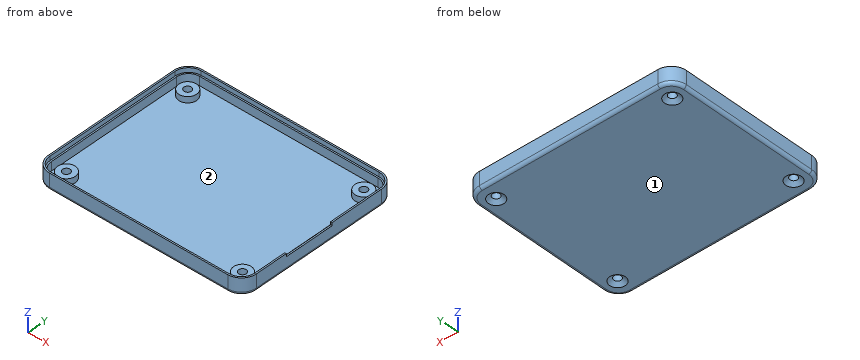
```python
from build123d import *

# Parameters (mm, degrees)
BOX012_W          = 69
BOX012_H          = 55
BOX012_DEPTH      = 1.5
FILLET004_R       = 4.6
CYLINDER005_R     = 1.25
CYLINDER005_DEPTH = 4
CYLINDER007_R     = 1.25
CYLINDER007_DEPTH = 4
CYLINDER009_R     = 1.25
CYLINDER009_DEPTH = 4
CYLINDER003_R     = 1.25
CYLINDER003_DEPTH = 4
BOX015_W          = 24
BOX015_H          = 16.8
BOX015_DEPTH      = 18
CYLINDER006_R     = 3
CYLINDER006_DEPTH = 3
CYLINDER008_R     = 3
CYLINDER008_DEPTH = 3
CYLINDER010_R     = 3
CYLINDER010_DEPTH = 3
BOX_W             = 68
BOX_H             = 54
BOX_DEPTH         = 4.5
FILLET006_R       = 4
THICKNESS_T       = 1
CYLINDER004_R     = 3
CYLINDER004_DEPTH = 3


with BuildPart() as snapbottom001:
    # Box012 → Box012 (new body)
    with BuildSketch(Plane(origin=(-0.5, -0.5, 3), x_dir=(1, 0, 0), z_dir=(0, 0, 1))):
        with Locations((34.5, 27.5)):
            Rectangle(BOX012_W, BOX012_H)
    extrude(amount=BOX012_DEPTH)

    # Fillet004
    fillet004_edges = [snapbottom001.edges().sort_by_distance(p)[0] for p in [
        (-0.5, -0.5, 3.75),
        (-0.5, 54.5, 3.75),
        (68.5, -0.5, 3.75),
        (68.5, 54.5, 3.75),
    ]]
    fillet(fillet004_edges, radius=FILLET004_R)


with BuildPart() as screwcone001:
    # Cone001 → Cone001 (revolve)
    with BuildSketch(Plane(origin=(4.5, 49.15, -2), x_dir=(1, 0, 0), z_dir=(0, -1, 0))):
        Polygon((0, 0), (4, 0), (1.25, 2), (0, 2), align=None)
    revolve(axis=Axis((4.5, 49.15, -2), (0, 0, 1)))


with BuildPart() as screwcone002:
    # Cone002 → Cone002 (revolve)
    with BuildSketch(Plane(origin=(63.75, 49.15, -2), x_dir=(1, 0, 0), z_dir=(0, -1, 0))):
        Polygon((0, 0), (4, 0), (1.25, 2), (0, 2), align=None)
    revolve(axis=Axis((63.75, 49.15, -2), (0, 0, 1)))


with BuildPart() as screwcone003:
    # Cone003 → Cone003 (revolve)
    with BuildSketch(Plane(origin=(63.75, 4.65, -2), x_dir=(1, 0, 0), z_dir=(0, -1, 0))):
        Polygon((0, 0), (4, 0), (1.25, 2), (0, 2), align=None)
    revolve(axis=Axis((63.75, 4.65, -2), (0, 0, 1)))


with BuildPart() as obj1:
    # Cylinder005 → Cylinder005 (new body)
    with BuildSketch(Plane(origin=(4.5, 49.15, -2), x_dir=(1, 0, 0), z_dir=(0, 0, 1))):
        Circle(CYLINDER005_R)
    extrude(amount=CYLINDER005_DEPTH)


with BuildPart() as obj2:
    # Cylinder007 → Cylinder007 (new body)
    with BuildSketch(Plane(origin=(63.75, 4.65, -2), x_dir=(1, 0, 0), z_dir=(0, 0, 1))):
        Circle(CYLINDER007_R)
    extrude(amount=CYLINDER007_DEPTH)


with BuildPart() as obj3:
    # Cylinder009 → Cylinder009 (new body)
    with BuildSketch(Plane(origin=(63.75, 49.15, -2), x_dir=(1, 0, 0), z_dir=(0, 0, 1))):
        Circle(CYLINDER009_R)
    extrude(amount=CYLINDER009_DEPTH)


with BuildPart() as obj4:
    # Cylinder003 → Cylinder003 (new body)
    with BuildSketch(Plane(origin=(4.5, 4.65, -2), x_dir=(1, 0, 0), z_dir=(0, 0, 1))):
        Circle(CYLINDER003_R)
    extrude(amount=CYLINDER003_DEPTH)


with BuildPart() as bottomscrewholes:
    # Cone → Cone (revolve)
    with BuildSketch(Plane(origin=(4.5, 4.65, -2), x_dir=(1, 0, 0), z_dir=(0, -1, 0))):
        Polygon((0, 0), (4, 0), (1.25, 2), (0, 2), align=None)
    revolve(axis=Axis((4.5, 4.65, -2), (0, 0, 1)))

    # Fusion001: union ScrewCone001, ScrewCone002, ScrewCone003, obj1, obj2, obj3, obj4
    add(screwcone001.part)
    add(screwcone002.part)
    add(screwcone003.part)
    add(obj1.part)
    add(obj2.part)
    add(obj3.part)
    add(obj4.part)


with BuildPart() as bottomholes:
    # Box015 → Box015 (new body)
    with BuildSketch(Plane(origin=(47, 15, 3.5), x_dir=(1, 0, 0), z_dir=(0, 0, 1))):
        with Locations((12, 8.4)):
            Rectangle(BOX015_W, BOX015_H)
    extrude(amount=BOX015_DEPTH)

    # Fusion007: union snapbottom001, BottomScrewHoles
    add(snapbottom001.part)
    add(bottomscrewholes.part)


with BuildPart() as obj5:
    # Cylinder006 → Cylinder006 (new body)
    with BuildSketch(Plane(origin=(4.5, 49.15, -1), x_dir=(1, 0, 0), z_dir=(0, 0, 1))):
        Circle(CYLINDER006_R)
    extrude(amount=CYLINDER006_DEPTH)


with BuildPart() as obj6:
    # Cylinder008 → Cylinder008 (new body)
    with BuildSketch(Plane(origin=(63.75, 4.65, -1), x_dir=(1, 0, 0), z_dir=(0, 0, 1))):
        Circle(CYLINDER008_R)
    extrude(amount=CYLINDER008_DEPTH)


with BuildPart() as obj7:
    # Cylinder010 → Cylinder010 (new body)
    with BuildSketch(Plane(origin=(63.75, 49.15, -1), x_dir=(1, 0, 0), z_dir=(0, 0, 1))):
        Circle(CYLINDER010_R)
    extrude(amount=CYLINDER010_DEPTH)


with BuildPart() as thickness:
    # Box → Box (new body)
    with BuildSketch(Plane.XY):
        with Locations((34, 27)):
            Rectangle(BOX_W, BOX_H)
    extrude(amount=BOX_DEPTH)

    # Fillet006
    fillet006_edges = [thickness.edges().sort_by_distance(p)[0] for p in [
        (0, 0, 2.25),
        (0, 54, 2.25),
        (68, 0, 2.25),
        (68, 54, 2.25),
    ]]
    fillet(fillet006_edges, radius=FILLET006_R)

    # Thickness
    thickness_openings = [thickness.faces().sort_by_distance(p)[0] for p in [
        (34, 27, 4.5),
    ]]
    offset(amount=THICKNESS_T, openings=thickness_openings)


with BuildPart() as bottom:
    # Cylinder004 → Cylinder004 (new body)
    with BuildSketch(Plane(origin=(4.5, 4.65, -1), x_dir=(1, 0, 0), z_dir=(0, 0, 1))):
        Circle(CYLINDER004_R)
    extrude(amount=CYLINDER004_DEPTH)

    # Fusion006: union obj5, obj6, obj7, Thickness
    add(obj5.part)
    add(obj6.part)
    add(obj7.part)
    add(thickness.part)

    # Cut003: cut BottomHoles
    add(bottomholes.part, mode=Mode.SUBTRACT)


solid = bottom.part
```
Input: part model. Units: mm. Frame: model coordinates. Face numbers are marked on the shaded views. Coordinates: 2 decimals unless noted, no trailing zeros. Order: outer loops, then holes, each group sorted by start corner. A loop starts at its lowest first (then second) coordinate and runs counter-clockwise, first axis right, second up. Notation, with made-up numbers: (-13, 50) - (9, 50) arc R10 ccw to (9, 59) - close; hole circle Ø2 at (77, 36.25). An arc over 180 degrees is marked (long way). Put each result on its own line as item: value.
1. Cut plane B-B on y = 16. Return the cut outline in (x, z), then the cut area to 3 significant figures.
Report:
outline: (-1, 0) arc R1 ccw to (0, -1) - (68, -1) arc R1 ccw to (69, 0) - (69, 3.5) - (68.5, 3.5) - (68.5, 3) - (68, 3) - (68, 0) - (0, 0) - (0, 3) - (-0.5, 3) - (-0.5, 4.5) - (-1, 4.5) - close
area: 76.6 mm2
2. Line query: line 1 along Y through (x, z) = (4.5, 1); line 2 along Y through (x, z) = (14.5, 4.2); line 3 along X through (y, z) = (50, 3.85). Output: solid intervals per line, ascending.
Report:
line 1: y = -1 to 0, 1.65 to 3.4, 5.9 to 7.65, 46.15 to 47.9, 50.4 to 52.15, 54 to 55
line 2: y = -1 to -0.5, 54.5 to 55
line 3: x = -1 to -0.5, 68.5 to 69
3. Contact query for flat-ended pins moving along their axis: pin 1 Ø6 at (x, y) = (28, 10.5) entering from +Z; pin 2 Ø3 at (x, y) = (5, 5.5) entering from +Z; pin 3 Ø1.6 at (y, z) = (23, 4) entering from +X. Output: stop coordinate, or through.
Report:
pin 1: stops at z = 0
pin 2: stops at z = 2
pin 3: stops at x = 69
4. Cut plane C-C on x = 12. Return the cut outline in (y, z), then the cut area to 3 significant figures.
Report:
outline: (-1, 0) arc R1 ccw to (0, -1) - (54, -1) arc R1 ccw to (55, 0) - (55, 4.5) - (54.5, 4.5) - (54.5, 3) - (54, 3) - (54, 0) - (0, 0) - (0, 3) - (-0.5, 3) - (-0.5, 4.5) - (-1, 4.5) - close
area: 63.1 mm2
5. Draft query along X for the marked faces 1 and 2. Return one class per face: pulls with the +X half, pulls with the -X half, needs draft (parallel to the pull), parting line crosses it, or undercut.
Report:
face 1: needs draft
face 2: undercut
6. Cut plane A-A on z = 0.75. State how many separate pieces and enclosed holes the cut face has, then the cut area to 3 significant figures.
Report:
separate pieces: 5
enclosed holes: 5
area: 334 mm2
